Verification items for the finished model (mm, model axes). Give positions to 0.01 mm unless a question says otherwise; leave off trailing zeros. Loops run counter-clockwise (first coordinate to the right, second up) from the corner with the lowest first, then second, coordinate; pieces in that order, holes last. Notation, with made-up numbers: (75, -26.5) - (119, -26.5) arc R31 ccw to (119, 9.5) - close; hole circle Ø11 at (-37, 12.5). An arc over 180 degrees is marked (long way). Use one line per item in the form item = value.
```python
from build123d import *

# Parameters (mm, degrees)
BOSS_EXTRUDE1_DEPTH = 0.8
FILLET1_R           = 2
FILLET2_R           = 5
SKETCH2_R           = 1.2
CUT_EXTRUDE1_DEPTH  = 23.249719099
SKETCH3_R           = 1.2
CUT_EXTRUDE2_DEPTH  = 23.249719099
SKETCH5_W           = 15
SKETCH5_H           = 2
CUT_EXTRUDE3_DEPTH  = 23.249719099
FILLET3_R           = 1


with BuildPart() as part:
    # Sketch1 → Boss-Extrude1 (new, symmetric)
    with BuildSketch(Plane(origin=(0, 0, 0), x_dir=(1, 0, 0), z_dir=(0, 1, 0))):
        with BuildLine():
            Line((11.716387939, 7), (-8.827016654, 7))
            ThreePointArc((-8.827016654, 7), (-20.7, 0), (-8.827016654, -7))
            Line((-8.827016654, -7), (11.716387939, -7))
            Line((11.716387939, -7), (11.716387939, 7))
        make_face()
    extrude(amount=BOSS_EXTRUDE1_DEPTH, both=True)

    # Fillet1
    fillet1_edges = [part.edges().sort_by_distance(p)[0] for p in [
        (11.716387939, 0, 7),
        (11.716387939, 0, -7),
    ]]
    fillet(fillet1_edges, radius=FILLET1_R)

    # Fillet2
    fillet2_edges = [part.edges().sort_by_distance(p)[0] for p in [
        (-8.827016654, 0, 7),
        (-8.827016654, 0, -7),
    ]]
    fillet(fillet2_edges, radius=FILLET2_R)

    # Sketch2 → Cut-Extrude1 (cut, through all)
    with BuildSketch(Plane(origin=(0, 0.8, 0), x_dir=(1, 0, 0), z_dir=(0, 1, 0))):
        with Locations(Location((-8.2, 0, 0), (0, 0, 270))):
            Circle(SKETCH2_R)
        with Locations(Location((-12.7, 4.5, 0), (0, 0, 270))):
            Circle(SKETCH2_R)
        with Locations(Location((-17.2, 0, 0), (0, 0, 270))):
            Circle(SKETCH2_R)
        with Locations(Location((-12.7, -4.5, 0), (0, 0, 270))):
            Circle(SKETCH2_R)
        with Locations(Location((-12.7, 0, 0), (0, 0, 270))):
            Circle(SKETCH2_R)
    extrude(amount=-CUT_EXTRUDE1_DEPTH, mode=Mode.SUBTRACT)

    # Sketch3 → Cut-Extrude2 (cut, through all)
    with BuildSketch(Plane(origin=(0, 0.8, 0), x_dir=(1, 0, 0), z_dir=(0, 1, 0))):
        with Locations(Location((9.121387939, 4.25, 0), (0, 0, 270))):
            Circle(SKETCH3_R)
        with Locations(Location((9.121387939, -4.25, 0), (0, 0, 270))):
            Circle(SKETCH3_R)
        with Locations(Location((6.871387939, 0, 0), (0, 0, 270))):
            Circle(SKETCH3_R)
    extrude(amount=-CUT_EXTRUDE2_DEPTH, mode=Mode.SUBTRACT)

    # Sketch5 → Cut-Extrude3 (cut, through all)
    with BuildSketch(Plane(origin=(0, 0.8, 0), x_dir=(1, 0, 0), z_dir=(0, 1, 0))):
        with Locations((-0.783612061, 4.8)):
            Rectangle(SKETCH5_W, SKETCH5_H)
        with Locations((-0.783612061, -4.8)):
            Rectangle(SKETCH5_W, SKETCH5_H)
    extrude(amount=-CUT_EXTRUDE3_DEPTH, mode=Mode.SUBTRACT)

    # Fillet3
    fillet3_edges = [part.edges().sort_by_distance(p)[0] for p in [
        (-8.283612061, 0, 5.8),
        (6.716387939, 0, 5.8),
        (6.716387939, 0, 3.8),
        (-8.283612061, 0, 3.8),
        (-8.283612061, 0, -3.8),
        (6.716387939, 0, -3.8),
        (6.716387939, 0, -5.8),
        (-8.283612061, 0, -5.8),
    ]]
    fillet(fillet3_edges, radius=FILLET3_R - 0.0001)  # a hair under: the kernel refuses the full size


solid = part.part
```
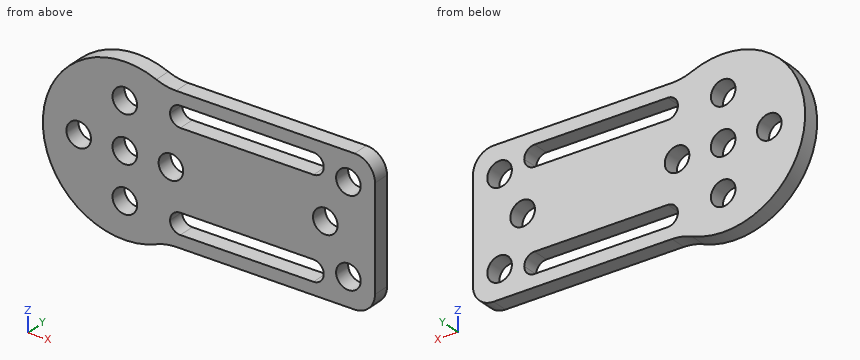
1. Section check A-A, the plane x = -12.7. Record the cut outline in (y, z), then the cut area to 3 significant figures.
Result set:
outline = (-0.8, -8) - (0.8, -8) - (0.8, -5.7) - (-0.8, -5.7) - close; (-0.8, -3.3) - (0.8, -3.3) - (0.8, -1.2) - (-0.8, -1.2) - close; (-0.8, 1.2) - (0.8, 1.2) - (0.8, 3.3) - (-0.8, 3.3) - close; (-0.8, 5.7) - (0.8, 5.7) - (0.8, 8) - (-0.8, 8) - close
area = 14.1 mm²
2. Section check B-B, the plane z = 0. Record the cut outline in (x, y), then the cut area to 3 significant figures.
Result set:
outline = (-20.7, -0.8) - (-18.4, -0.8) - (-18.4, 0.8) - (-20.7, 0.8) - close; (-16, -0.8) - (-13.9, -0.8) - (-13.9, 0.8) - (-16, 0.8) - close; (-11.5, -0.8) - (-9.4, -0.8) - (-9.4, 0.8) - (-11.5, 0.8) - close; (-7, -0.8) - (5.67, -0.8) - (5.67, 0.8) - (-7, 0.8) - close; (8.07, -0.8) - (11.72, -0.8) - (11.72, 0.8) - (8.07, 0.8) - close
area = 36.5 mm²
3. Section check D-D, the plane x = -9. Record the cut outline in (y, z), then the cut area to 3 significant figures.
Result set:
outline = (-0.8, -7.17) - (0.8, -7.17) - (0.8, -0.89) - (-0.8, -0.89) - close; (-0.8, 0.89) - (0.8, 0.89) - (0.8, 7.17) - (-0.8, 7.17) - close
area = 20.1 mm²
4. Scan lines: probe 1 along Z at (x, y) = (3, 0.25); probe 2 along X at (y, z) = (0.25, 0); probe 3 along X at (y, z) = (0.55, -4.5). Record each from-to range of solid material in increasing order.
Result set:
probe_1 = -7 to -5.8, -3.8 to 3.8, 5.8 to 7
probe_2 = -20.7 to -18.4, -16 to -13.9, -11.5 to -9.4, -7 to 5.67, 8.07 to 11.72
probe_3 = -19.31 to -13.9, -11.5 to -8.24, 6.67 to 7.95, 10.3 to 11.72
5. Section check C-C, the plane y = -0.15. State how many separate pieces and enclosed holes the cut face has, then the cut area to 3 significant figures.
Result set:
separate_pieces = 1
enclosed_holes = 10
area = 352 mm²
6. Depth check by flat-ended pin: pin 1 Ø0.8 at (x, y) = (0, 0) entering from +Z; pin 2 Ø0.8 at (x, y) = (-2, 0) entering from -Z. Enter the tip coordinate at first touch or a pass-through.
Result set:
pin_1 = 7
pin_2 = -7
